```python
from build123d import *

# Parameters (mm, degrees)
SALIENTE_EXTRUIR1_DEPTH     = 2
CROQUIS2_W                  = 13.9
CROQUIS2_H                  = 20
SALIENTE_EXTRUIR2_DEPTH     = 24.5
SALIENTE_EXTRUIR3_DEPTH     = 22.5
CROQUIS5_R                  = 2.1
CORTAR_EXTRUIR2_DEPTH       = 20.5
CROQUIS16_W                 = 3
CROQUIS16_H                 = 33.930468167
CORTAR_EXTRUIR8_DEPTH       = 22.5
CORTAR_EXTRUIR1_DEPTH       = 27
CORTAR_EXTRUIR1_DEPTH_BACK  = 65.5
CROQUIS4_R                  = 1.599999999
REDONDEO1_R                 = 3
REDONDEO2_R                 = 5
SALIENTE_EXTRUIR5_START     = 2
SALIENTE_EXTRUIR5_DEPTH     = 2
REDONDEO6_R                 = 2
REDONDEO7_R                 = 2
CROQUIS17_R                 = 2.1
CORTAR_EXTRUIR9_DEPTH       = 10
CORTAR_EXTRUIR14_DEPTH      = 11
CORTAR_EXTRUIR14_DEPTH_BACK = 10
CROQUIS18_R                 = 1.9
CROQUIS19_R                 = 18.5
CORTAR_EXTRUIR15_DEPTH      = 3.5
CORTAR_EXTRUIR16_START      = -56
CROQUIS20_R                 = 18.5
CORTAR_EXTRUIR16_DEPTH      = 3.5
CORTAR_EXTRUIR17_DEPTH      = 47
CORTAR_EXTRUIR17_DEPTH_BACK = 86
CROQUIS21_W                 = 7.397871061
CROQUIS21_H                 = 19.885366365


# Some blends are built 0.0001 mm under size
with BuildPart() as part:
    # Croquis1 → Saliente-Extruir1 (new body)
    with BuildSketch(Plane(origin=(0, 0, 0), x_dir=(1, 0, 0), z_dir=(0, 1, 0))):
        with BuildLine():
            Line((-31.5, -9.464532567), (31.5, -9.464532567))
            Line((31.5, -9.464532567), (31.5, 7.964532567))
            ThreePointArc((31.5, 7.964532567), (31.060660172, 9.025192739), (30, 9.464532567))
            Line((30, 9.464532567), (28.160101256, 9.464532567))
            ThreePointArc((28.160101256, 9.464532567), (27.099441084, 9.903872396), (26.660101256, 10.964532567))
            Line((26.660101256, 10.964532567), (26.660101256, 14.266885585))
            ThreePointArc((26.660101256, 14.266885585), (20.802236879, 28.409021208), (6.660101256, 34.266885585))
            Line((6.660101256, 34.266885585), (-6.660101256, 34.266885585))
            ThreePointArc((-6.660101256, 34.266885585), (-20.802236879, 28.409021208), (-26.660101256, 14.266885585))
            Line((-26.660101256, 14.266885585), (-26.660101256, 10.964532567))
            ThreePointArc((-26.660101256, 10.964532567), (-27.099441084, 9.903872396), (-28.160101256, 9.464532567))
            Line((-28.160101256, 9.464532567), (-30, 9.464532567))
            ThreePointArc((-30, 9.464532567), (-31.060660172, 9.025192739), (-31.5, 7.964532567))
            Line((-31.5, 7.964532567), (-31.5, -9.464532567))
        make_face()
    extrude(amount=SALIENTE_EXTRUIR1_DEPTH)

    # Croquis2 → Saliente-Extruir2 (add)
    with BuildSketch(Plane(origin=(0, 0, 0), x_dir=(1, 0, 0), z_dir=(0, 1, 0))):
        Rectangle(CROQUIS2_W, CROQUIS2_H)
    extrude(amount=SALIENTE_EXTRUIR2_DEPTH)

    # Croquis3 → Saliente-Extruir3 (add)
    with BuildSketch(Plane(origin=(0, 2, 0), x_dir=(1, 0, 0), z_dir=(0, 1, 0))):
        with BuildLine():
            ThreePointArc((28.160101256, 9.464532567), (27.375457574, 9.686121721), (26.822638598, 10.285420177))
            Line((26.822638598, 10.285420177), (25.6, 10.285420177))
            Line((25.6, 10.285420177), (25.6, -2.749999823))
            Line((25.6, -2.749999823), (31.5, -2.749999823))
            Line((31.5, -2.749999823), (31.5, 7.964532567))
            ThreePointArc((31.5, 7.964532567), (31.060660172, 9.025192739), (30, 9.464532567))
            Line((30, 9.464532567), (28.160101256, 9.464532567))
        make_face()
        with BuildLine():
            Line((-25.6, 10.285420177), (-26.822638598, 10.285420177))
            ThreePointArc((-26.822638598, 10.285420177), (-27.375457574, 9.686121721), (-28.160101256, 9.464532567))
            Line((-28.160101256, 9.464532567), (-30, 9.464532567))
            ThreePointArc((-30, 9.464532567), (-31.060660172, 9.025192739), (-31.5, 7.964532567))
            Line((-31.5, 7.964532567), (-31.5, -2.749999823))
            Line((-31.5, -2.749999823), (-25.6, -2.749999823))
            Line((-25.6, -2.749999823), (-25.6, 10.285420177))
        make_face()
    extrude(amount=SALIENTE_EXTRUIR3_DEPTH)

    # Croquis5 → Cortar-Extruir2 (cut)
    with BuildSketch(Plane(origin=(0, 24.5, 0), x_dir=(1, 0, 0), z_dir=(0, 1, 0))):
        with Locations(Location((0, 1.798301608, 0), (0, 0, 270))):
            Circle(CROQUIS5_R)
        with Locations(Location((0, -6.026932469, 0), (0, 0, 270))):
            Circle(CROQUIS5_R)
        with Locations(Location((-28.55, 1.798301608, 0), (0, 0, 270))):
            Circle(CROQUIS5_R)
        with Locations(Location((28.55, 1.798301608, 0), (0, 0, 270))):
            Circle(CROQUIS5_R)
    extrude(amount=-CORTAR_EXTRUIR2_DEPTH, mode=Mode.SUBTRACT)

    # Croquis16 → Cortar-Extruir8 (cut)
    with BuildSketch(Plane(origin=(0, 24.5, 0), x_dir=(1, 0, 0), z_dir=(0, 1, 0))):
        with Locations((5.45, 0.270579682)):
            Rectangle(CROQUIS16_W, CROQUIS16_H)
        with Locations((-5.45, 0.270579682)):
            Rectangle(CROQUIS16_W, CROQUIS16_H)
    extrude(amount=-CORTAR_EXTRUIR8_DEPTH, mode=Mode.SUBTRACT)

    # Croquis4 → Cortar-Extruir1 (cut, two sides: drawn at the far end of the back side and taken through both)
    with BuildSketch(Plane.ZY.offset(25.5).offset(-CORTAR_EXTRUIR1_DEPTH_BACK)):
        with Locations(Location((-6.002353017, 4.3, 0), (0, 0, 180))):
            Circle(CROQUIS4_R)
        with Locations(Location((-6.002353017, 22.4, 0), (0, 0, 180))):
            Circle(CROQUIS4_R)
    extrude(amount=CORTAR_EXTRUIR1_DEPTH + CORTAR_EXTRUIR1_DEPTH_BACK, mode=Mode.SUBTRACT)

    # Redondeo1
    # the kernel refuses this fillet: 3 mm, written as the material it adds along each edge
    with BuildSketch(Plane(origin=(25.6, 2, 2.749999823), x_dir=(0, 0, 1), z_dir=(1, 0, 0))) as redondeo1_piece_1:
        with BuildLine():
            CenterArc((REDONDEO1_R, -REDONDEO1_R), REDONDEO1_R, 90, 90)
            Line((0, -REDONDEO1_R), (0, 0))
            Line((0, 0), (REDONDEO1_R, 0))
        make_face()
    extrude(amount=5.9)
    # the kernel refuses this fillet: 3 mm, written as the material it takes off along each edge
    with BuildSketch(Plane(origin=(11.45, 24.5, 10), x_dir=(0, 0, -1), z_dir=(-1, 0, 0))) as redondeo1_2_piece_1:
        with BuildLine():
            CenterArc((REDONDEO1_R, REDONDEO1_R), REDONDEO1_R, 180, 90)
            Line((0, REDONDEO1_R), (0, 0))
            Line((0, 0), (REDONDEO1_R, 0))
        make_face()
    extrude(amount=22.9, mode=Mode.SUBTRACT)

    # Redondeo2
    redondeo2_edges = [part.edges().sort_by_distance(p)[0] for p in [
        (0, 2, -10),
    ]]
    fillet(redondeo2_edges, radius=REDONDEO2_R)

    # Croquis15 → Saliente-Extruir5 (add)
    with BuildSketch(Plane.XZ.offset(SALIENTE_EXTRUIR5_START)):
        with BuildLine():
            Line((-31.5, 9.464532567), (31.5, 9.464532567))
            Line((31.5, 9.464532567), (31.5, -7.489095092))
            ThreePointArc((31.5, -7.489095092), (30.914213562, -8.903308654), (29.5, -9.489095092))
            Line((29.5, -9.489095092), (28.660101256, -9.489095092))
            ThreePointArc((28.660101256, -9.489095092), (27.245887693, -10.074881529), (26.660101256, -11.489095092))
            Line((26.660101256, -11.489095092), (26.660101256, -14.266885585))
            ThreePointArc((26.660101256, -14.266885585), (20.802236879, -28.409021208), (6.660101256, -34.266885585))
            Line((6.660101256, -34.266885585), (1.137553535, -34.266885585))
            Line((1.137553535, -34.266885585), (-1.137553535, -34.266885585))
            Line((-1.137553535, -34.266885585), (-6.660101256, -34.266885585))
            ThreePointArc((-6.660101256, -34.266885585), (-20.802236879, -28.409021208), (-26.660101256, -14.266885585))
            Line((-26.660101256, -14.266885585), (-26.660101256, -11.489095092))
            ThreePointArc((-26.660101256, -11.489095092), (-27.245887693, -10.074881529), (-28.660101256, -9.489095092))
            Line((-28.660101256, -9.489095092), (-29.5, -9.489095092))
            ThreePointArc((-29.5, -9.489095092), (-30.914213562, -8.903308654), (-31.5, -7.489095092))
            Line((-31.5, -7.489095092), (-31.5, 9.464532567))
        make_face()
    extrude(amount=-SALIENTE_EXTRUIR5_DEPTH)

    # Redondeo6
    redondeo6_edges = [part.edges().sort_by_distance(p)[0] for p in [
        (-31.5, -2, 0.987718738),
        (-30.914213562, -2, -8.903308654),
        (-29.080050628, -2, -9.489095092),
        (-27.245887693, -2, -10.074881529),
        (-26.660101256, -2, -12.877990338),
        (-20.802236879, -2, -28.409021208),
        (0, -2, -34.266885585),
        (20.802236879, -2, -28.409021208),
        (26.660101256, -2, -12.877990338),
        (27.245887693, -2, -10.074881529),
        (29.080050628, -2, -9.489095092),
        (30.914213562, -2, -8.903308654),
        (31.5, -2, 0.987718738),
    ]]
    fillet(redondeo6_edges, radius=REDONDEO6_R - 0.0001)  # a hair under: the kernel refuses the full size

    # Redondeo7
    redondeo7_edges = [part.edges().sort_by_distance(p)[0] for p in [
        (31.5, 0.99995, 9.464532567),
        (-31.5, 0.99995, 9.464532567),
        (0, -2, 9.464532567),
        (30.914242852, -1.414242852, 9.464532567),
        (-30.914242852, -1.414242852, 9.464532567),
    ]]
    fillet(redondeo7_edges, radius=REDONDEO7_R - 0.0001)  # a hair under: the kernel refuses the full size

    # Croquis17 → Cortar-Extruir9 (cut, symmetric)
    with BuildSketch(Plane(origin=(0, 0, 0), x_dir=(0, 0, -1), z_dir=(1, 0, 0))):
        with Locations((6.002353017, 4.3)):
            Circle(CROQUIS17_R)
    extrude(amount=CORTAR_EXTRUIR9_DEPTH, both=True, mode=Mode.SUBTRACT)

    # Croquis18 → Cortar-Extruir14 (cut, two sides: drawn at the far end of the back side and taken through both)
    with BuildSketch(Plane(origin=(0, 0, 0), x_dir=(0, 0, -1), z_dir=(1, 0, 0)).offset(-CORTAR_EXTRUIR14_DEPTH_BACK)):
        with Locations((6.002353017, 22.4)):
            Circle(CROQUIS18_R)
    extrude(amount=CORTAR_EXTRUIR14_DEPTH + CORTAR_EXTRUIR14_DEPTH_BACK, mode=Mode.SUBTRACT)

    # Croquis19 → Cortar-Extruir15 (cut)
    with BuildSketch(Plane(origin=(31.5, 0, 0), x_dir=(0, 0, -1), z_dir=(1, 0, 0))):
        with Locations((25.179802512, 14.045485316)):
            Circle(CROQUIS19_R)
    extrude(amount=-CORTAR_EXTRUIR15_DEPTH, mode=Mode.SUBTRACT)

    # Croquis20 → Cortar-Extruir16 (cut)
    with BuildSketch(Plane(origin=(28, 0, 0), x_dir=(0, 0, -1), z_dir=(1, 0, 0)).offset(CORTAR_EXTRUIR16_START)):
        with Locations((25.179802512, 14.045485316)):
            Circle(CROQUIS20_R)
    extrude(amount=-CORTAR_EXTRUIR16_DEPTH, mode=Mode.SUBTRACT)

    # Croquis21 → Cortar-Extruir17 (cut, two sides: drawn at the far end of the back side and taken through both)
    with BuildSketch(Plane(origin=(0, 2, 0), x_dir=(1, 0, 0), z_dir=(0, 1, 0)).offset(-CORTAR_EXTRUIR17_DEPTH_BACK)):
        with Locations((-28.769498571, 0.478150615)):
            Rectangle(CROQUIS21_W, CROQUIS21_H)
        with Locations((28.769498571, 0.478150615)):
            Rectangle(CROQUIS21_W, CROQUIS21_H)
    extrude(amount=CORTAR_EXTRUIR17_DEPTH + CORTAR_EXTRUIR17_DEPTH_BACK, mode=Mode.SUBTRACT)


solid = part.part
```
Design review of the part built by this model. Coordinates are the model's own, in mm. A direction names the side the tool comes from. Coordinates: 2 decimals unless noted, no trailing zeros. Order: outer loops, then holes, each group sorted by start corner. A loop starts at its lowest first (then second) coordinate and runs counter-clockwise, first axis right, second up.
1) Wall thickness on line 1 along Y through (x, z) = (-15, -7); line 2 along Z through (x, y) = (1.5, 22.4); line 3 along X through (y, z) = (21, 0): over which ranges is each line inside the solid? List them lowest first.
2) Take a section at A-A, the plane y = 22.4. Give the boundary of the cut face in (x, z).
3) Mouldability with a two-part tool opening along Z and no side actions: class faces 4 (the flat face through (25.071, 0, 0)), 5 (the cylindrical face through (-0.055, 20.714, -6.879)), 6 (the cylindrical face through (-20.65, 0.99, -28.56)) as +Z half, -Z half, draft (parallel to the pull), parting line (faces both ways), or undercut.
4) Clearance check with flat-ended pins moving along their axes: pin 1 (5 mm diameter, centred on x = -14, z = -27.5, fed in from +Y); pin 2 (0.6 mm diameter, centred on x = -26, y = 0, fed in from +Z); pin 3 (2.5 mm diameter, centred on x = 0, z = -1.8, fed in from +Y). State where each tip first meets the part, or that it passes through.
5) Take a section at C-C, the plane z = 2. Give the boundary of the cut face in (x, y).
6) For faces 1 (the cylindrical face through (26.06, -1.43, -12.9)), 2 (the cylindrical face through (0.631, 14.394, 0.205)), 3 (the flat face through (3.95, 13, 0)), list the 3-axis set-ups (+Z, -Z, +X, -X, +Y, -Y) from which the entire face can be reached by the end or side of a thin tool; tool diameter is ignored.
7) Take a section at B-B, the plane x = 0. State how many separate pieces and enclosed holes the cut face has, and give its area (3 significant figures).
Returned:
1. line 1: y = -2 to 2
1. line 2: z = -10 to -7.9, -4.1 to -3.27, -0.33 to 4.56, 7.5 to 9.86
1. line 3: x = -3.95 to -1.08, 1.08 to 3.95
2. outline: (-3.95, -10) - (3.95, -10) - (3.95, -7.9) - (-3.95, -7.9) - close; (-3.95, -4.1) - (3.95, -4.1) - (3.95, 9.86) - (-3.95, 9.86) - close; hole circle Ø4.2 at (0, -1.8); hole circle Ø4.2 at (0, 6.03)
3. face 4: draft
3. face 5: undercut
3. face 6: -Z half
4. pin 1: stops at y = 2
4. pin 2: stops at z = -10.42
4. pin 3: stops at y = 4
5. outline: (-25.07, -2) - (25.07, -2) - (25.07, 2) - (3.95, 2) - (3.95, 24.5) - (-3.95, 24.5) - (-3.95, 2) - (-25.07, 2) - close
6. face 1: -Z, +X, -Y
6. face 2: +Y
6. face 3: +Z, -Z, +X, +Y
7. separate pieces: 1
7. enclosed holes: 2
7. area: 430 mm2
